Can you work these out from the model? Positions are in its coordinate system, mm. Face numbers are marked on the shaded views. Round coordinates to 2 decimals unless told otherwise and drop trailing zeros. Write each loop counter-clockwise with the first axis right and the second up, starting at its lowest first coordinate (ties: lowest second). Pieces come first, ordered by that corner, then holes. Notation, with made-up numbers: M 47,-35.75 L 52,-35.75 A26 cw 52,-19.75 Z; hole C 1,-22.75 d7. An arc over 180 degrees is marked long. Answer in a Markdown table with one row per item. Add a question column.
(1) If we mould it in two halves opening along X, with no side actions, what happens to the marked faces 1, 2 and 3? For each: released by +X, released by -X, zero draft, split by the parting line, or undercut.
(2) Suppose I cut it at D-D, the plane y = 9.25. Write out the boundary of the cut face in (x, z), then the cut area to 3 significant figures.
(3) I'm going to push flat-ended pins straight in: pin 1 (6 mm diameter, centred on y = 14, z = -1, fed in from +X); pin 2 (4 mm diameter, centred on x = 7.5, y = 10.5, fed in from -Z); pin 3 (2 mm diameter, centred on y = 10.5, z = -16, fed in from +X); pin 4 (1 mm diameter, centred on y = 12.5, z = 5, fed in from +X). Where does each tip first touch, or does it pass through?
(4) If I drill on probe 1 along Z at (x, y) = (0, 18); probe 2 along X at (y, z) = (6.5, 5); probe 3 along Z at (x, y) = (3.5, 7), over which ranges is the centre line in solid material (lowest first)?
(5) Suppose I cut it at C-C, the plane y = 18. Write out the boundary of the cut face in (x, z), then the cut area to 3 significant figures.
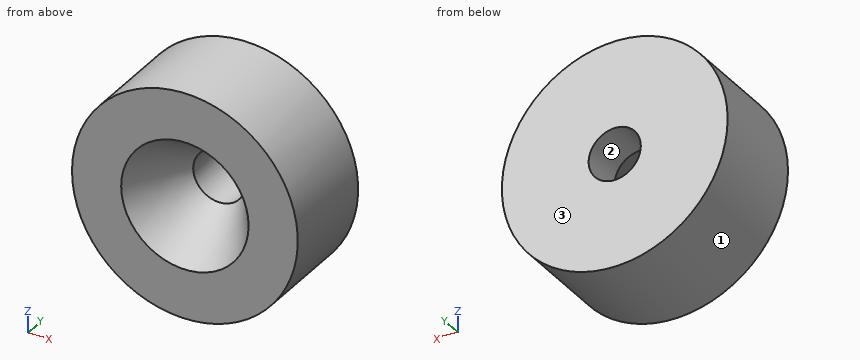
Autodesk Inventor part; units mm, degrees
ref_plane "YZ Plane" through (0, 0, 0) normal (1, 0, 0) x (0, 1, 0)
ref_plane "XZ Plane" through (0, 0, 0) normal (0, 1, 0) x (-1, 0, 0)
ref_plane "XY Plane" through (0, 0, 0) normal (0, 0, 1) x (1, 0, 0)
sketch "Sketch1" plane through (0, 0, 0) normal (0, 1, 0) x (-1, 0, 0)
  circle A0 centre (0, 0) radius 22.5
  circle A1 centre (0, 0) radius 12.7
  circle A2 centre (0, 0) radius 5.2
  dimension "d1" = 45
  dimension "d14" = 25.4
  dimension "d15" = 10.4
extrude "Extrusion1" add sketch "Sketch1" along normal blind 20 contours A0 | A1 | A2
extrude "Extrusion2" cut sketch "Sketch1" along normal blind 11.4 contours A1
extrude "Extrusion3" cut sketch "Sketch1" along normal blind 20 contours A2
chamfer "Chamfer2" distance 11.4 distance2 7.5 1 edges at (12.7, 11.4, 0) measured on face at (-12.5355, 7.6, -2.0372)
properties part number "4. ring"
Calculated:
| question | item | result |
|---|---|---|
| 1 | face 1 | split by the parting line |
| 1 | face 2 | undercut |
| 1 | face 3 | zero draft |
| 2 | outline | C 0,0 d45; hole C 0,0 d13.23 |
| 2 | area | 1,450 mm² |
| 3 | pin 1 | x = 22.5 |
| 3 | pin 2 | z = -21.82 |
| 3 | pin 3 | x = 16.77 |
| 3 | pin 4 | x = 22.05 |
| 4 | probe 1 | -22.5 to -5.2, 5.2 to 22.5 |
| 4 | probe 2 | -21.94 to -6.78, 6.78 to 21.94 |
| 4 | probe 3 | -22.23 to -7.3, 7.3 to 22.23 |
| 5 | outline | C 0,0 d45; hole C 0,0 d10.4 |
| 5 | area | 1,510 mm² |
